The drawing under review shows one solid part. Ordinate dimensions are in mm from its lowest x, y, z. A direction names the side the tool comes from. Round coordinates to 2 decimals unless told otherwise and drop trailing zeros. Loops run counter-clockwise (first coordinate to the right, second up) from the corner with the lowest first, then second, coordinate; pieces in that order, holes last. Notation, with made-up numbers: (30.25, 57) - (87.25, 57) arc R21 cw to (87.25, 70) - close; hole circle Ø5 at (-6, 33). An arc over 180 degrees is marked (long way). Answer as CSV lines item,"result".
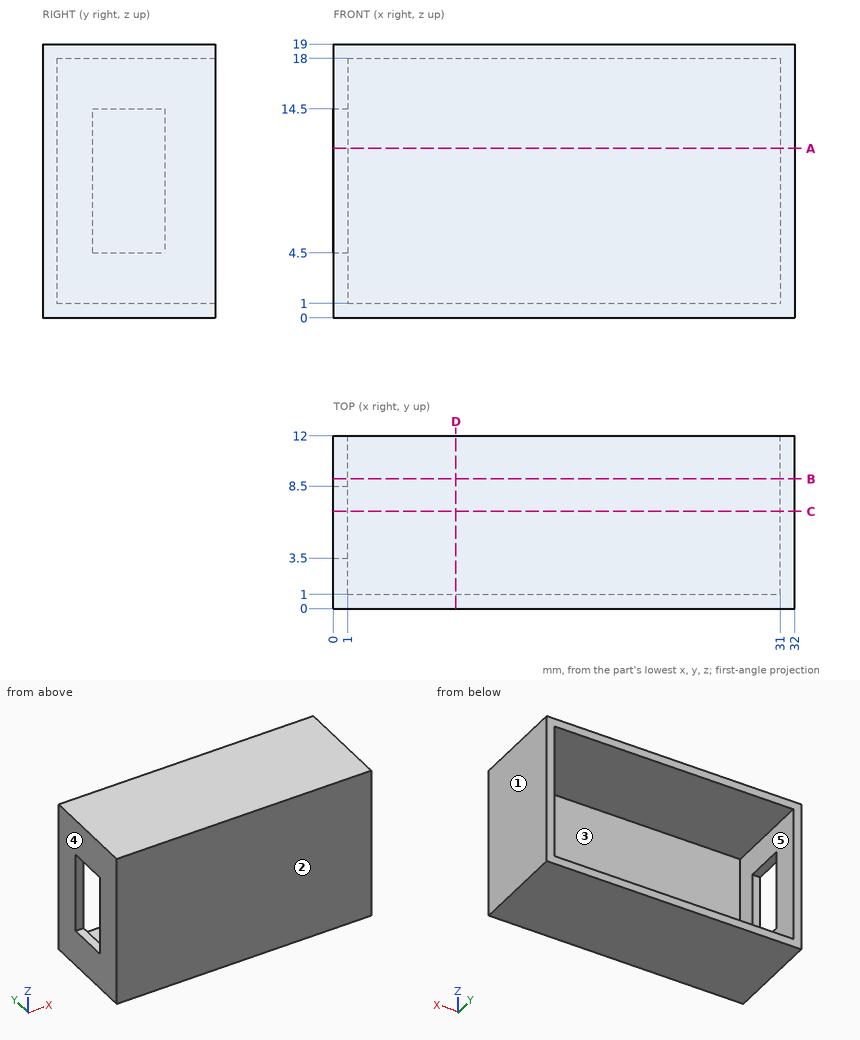
1. Tool access review of the marked faces 4 and 5: name each direction out of +Z, -Z, +X, -X, +Y, -Y from which nothing blocks a thin tool from reaching the whole face with its end or side.
Numbers:
face 4,"+Z, -Z, -X, +Y, -Y"
face 5,"+Y"
2. Take a section at D-D (x = 8.5). State the section outline as (y, z) points.
Numbers:
outline,"(0, 0) - (12, 0) - (12, 1) - (1, 1) - (1, 18) - (12, 18) - (12, 19) - (0, 19) - close"
3. Take a section at A-A (z = 11.75). State the section outline as (x, y) points, plus the area to 3 significant figures.
Numbers:
outline,"(0, 0) - (32, 0) - (32, 12) - (31, 12) - (31, 1) - (1, 1) - (1, 3.5) - (0, 3.5) - close; (0, 8.5) - (1, 8.5) - (1, 12) - (0, 12) - close"
area,"49.0 mm²"
4. Clearance check with flat-ended pins moving along their axes: pin 1 (2 mm diameter, centred on x = 13.5, y = 4.5, fed in from -Z); pin 2 (1 mm diameter, centred on x = 14.5, z = 11, fed in from +Y). State where each tip first meets the part, or that it passes through.
Numbers:
pin 1,"stops at z = 0"
pin 2,"stops at y = 1"
5. Take a section at C-C (y = 6.75). State the section outline as (x, z) points, plus the area to 3 significant figures.
Numbers:
outline,"(0, 0) - (32, 0) - (32, 19) - (0, 19) - (0, 14.5) - (1, 14.5) - (1, 18) - (31, 18) - (31, 1) - (1, 1) - (1, 4.5) - (0, 4.5) - close"
area,"88.0 mm²"
6. Draft analysis for pull direction X (two halves, no side actions). For the marked faces 1, 2 and 3, state which applies: +X half, -X half, draft (parallel to the pull), parting line (faces both ways), or undercut.
Numbers:
face 1,"+X half"
face 2,"draft"
face 3,"undercut"
7. Take a section at B-B (y = 9). State the section outline as (x, z) points, plus the area to 3 significant figures.
Numbers:
outline,"(0, 0) - (32, 0) - (32, 19) - (0, 19) - close; hole (1, 1) - (31, 1) - (31, 18) - (1, 18) - close"
area,"98.0 mm²"
8. Wall thickness on probe 1 along X at (y, z) = (3.75, 17.25); probe 2 along Z at (x, y) = (30.5, 5.75); probe 3 along Y at (x, z) = (15, 2.5): over which ranges is each line inside the solid? List them lowest first.
Numbers:
probe 1,"x = 0 to 1, 31 to 32"
probe 2,"z = 0 to 1, 18 to 19"
probe 3,"y = 0 to 1"
